Could you check a few things on this model? Use its own coordinates, in mm. A direction names the side the tool comes from. Round coordinates to 2 decimals unless told otherwise and drop trailing zeros. Loops run counter-clockwise (first coordinate to the right, second up) from the corner with the lowest first, then second, coordinate; pieces in that order, holes last. Notation, with made-up numbers: (-26.75, -33.75) - (-11.75, -33.75) arc R14 cw to (-11.75, -10.75) - close; hole circle Ø3 at (54.5, 28). An arc over 180 degrees is marked (long way). Answer as CSV lines item,"result". Start each with the question number.
1) We'd pull the mould along Z, two halves only. Please class faces 1 (the face through (0, -6.6, -6.1)), 2 (the face through (-2.17, -0.48, -7.53)), 3 (the face through (-5.714, 3.28, 18.811)): pulls with the +Z half, pulls with the -Z half, needs draft (parallel to the pull), parting line crosses it, or undercut.
2) Suppose I cut it at B-B, the plane z = -2.5. Write out the boundary of the cut face in (x, y), then the cut area to 3 significant figures.
3) I'm going to push flat-ended pins straight in: pin 1 Ø1.5 at (x, z) = (4, 10.5) entering from -Y; pin 2 Ø6 at (x, z) = (4.5, 4.5) entering from +Y; pin 3 Ø3 at (x, z) = (5, -13) entering from -Y; pin 4 Ø1.2 at (x, y) = (-1, 0) entering from +Z. Where does each tip first touch, or does it pass through?
4) Please list where these lines run through material, in increasing order: line 1 along Y through (x, z) = (0, 13.75); line 2 along Z through (x, y) = (2.25, 4); line 3 along Z through (x, y) = (1.5, -0.75).
5) Suppose I cut it at A-A, the plane z = 16.5. Write out the boundary of the cut face in (x, y).
6) Which directions (+Z, -Z, +X, -X, +Y, -Y) give clear straight access to the entire face, cutting with the end or side of a thin tool? Please do faces 4 (the face through (-5.7, 3.31, -6.11)), 5 (the face through (1.987, 0.626, 13.572)), 6 (the face through (3, 0, -6.35)), 7 (the face through (5.714, -3.28, 18.811)), 8 (the face through (-3.1, -0.69, -13.87)).
```python
from build123d import *

# Parameters (mm, degrees)
BOSS_EXTRUDE1_START = 19.05
BOSS_EXTRUDE1_DEPTH = 25.4
CHAMFER1_SIZE       = 0.9525
SKETCH4_R           = 2.0828
CUT_EXTRUDE1_DEPTH  = 11.1125
FILLET1_R           = 0.09921875
SKETCH5_OUTSIDE_W   = 101.45
SKETCH5_OUTSIDE_H   = 103.414
SKETCH5_OUTSIDE_R   = 6.35
CUT_EXTRUDE2_DEPTH  = 39.1
CUT_EXTRUDE2_TAPER  = 45
SKETCH6_OUTSIDE_W   = 76.05
SKETCH6_OUTSIDE_H   = 78.014
SKETCH6_OUTSIDE_R   = 6.35
CUT_EXTRUDE3_DEPTH  = 26.4
CUT_EXTRUDE3_TAPER  = 45


with BuildPart() as part:
    # Sketch2 → Boss-Extrude1 (new body)
    with BuildSketch(Plane.XY.offset(BOSS_EXTRUDE1_START)):
        Polygon((6.35, 3.666174209), (0, 7.332348419), (-6.35, 3.666174209), (-6.35, -3.666174209), (0, -7.332348419), (6.35, -3.666174209), align=None)
    extrude(amount=-BOSS_EXTRUDE1_DEPTH)

    # Sketch3 → Revolve1 (revolve)
    with BuildSketch(Plane(origin=(0, 0, 0), x_dir=(0, 0, -1), z_dir=(1, 0, 0))):
        Polygon((6.35, 2.2225), (8.5725, 2.2225), (9.525, 3.175), (19.05, 3.175), (19.05, 0), (6.35, 0), align=None)
    revolve(axis=Axis((0, 0, 19.05), (0, 0, -1)))

    # Chamfer1
    chamfer1_edges = [part.edges().sort_by_distance(p)[0] for p in [
        (0, -3.175, -19.05),
    ]]
    chamfer(chamfer1_edges, length=CHAMFER1_SIZE)

    # Sketch4 → Cut-Extrude1 (cut)
    with BuildSketch(Plane.XY.offset(19.05)):
        Circle(SKETCH4_R)
    extrude(amount=-CUT_EXTRUDE1_DEPTH, mode=Mode.SUBTRACT)

    # Fillet1
    fillet1_edges = [part.edges().sort_by_distance(p)[0] for p in [
        (0, -2.2225, -6.35),
    ]]
    fillet(fillet1_edges, radius=FILLET1_R)

    # Sketch5 outside → Cut-Extrude2 (cut, through all)
    with BuildSketch(Plane.XY.offset(19.05)):
        Rectangle(SKETCH5_OUTSIDE_W, SKETCH5_OUTSIDE_H)
        Circle(SKETCH5_OUTSIDE_R, mode=Mode.SUBTRACT)
    extrude(amount=-CUT_EXTRUDE2_DEPTH, taper=CUT_EXTRUDE2_TAPER, mode=Mode.SUBTRACT)

    # Sketch6 outside → Cut-Extrude3 (cut, through all)
    with BuildSketch(Plane(origin=(0, 0, -6.35), x_dir=(-1, 0, 0), z_dir=(0, 0, -1))):
        Rectangle(SKETCH6_OUTSIDE_W, SKETCH6_OUTSIDE_H)
        Circle(SKETCH6_OUTSIDE_R, mode=Mode.SUBTRACT)
    extrude(amount=-CUT_EXTRUDE3_DEPTH, taper=CUT_EXTRUDE3_TAPER, mode=Mode.SUBTRACT)


solid = part.part
```
Filled sheet:
1,face 1,"pulls with the -Z half"
1,face 2,"undercut"
1,face 3,"pulls with the +Z half"
2,outline,"(-6.35, -3.67) - (0, -7.33) - (6.35, -3.67) - (6.35, 3.67) - (0, 7.33) - (-6.35, 3.67) - close"
2,area,"140 mm²"
3,pin 1,"y = -5.46"
3,pin 2,"y = 6.47"
3,pin 3,"through"
3,pin 4,"z = 7.94"
4,line 1,"-7.33 to -2.08, 2.08 to 7.33"
4,line 2,"-6.35 to 19.05"
4,line 3,"-19.05 to 7.94"
5,outline,"(-6.35, -3.67) - (0, -7.33) - (6.35, -3.67) - (6.35, 3.67) - (0, 7.33) - (-6.35, 3.67) - close; hole circle Ø4.17 at (0, 0)"
6,face 4,"-Z, -X, +Y"
6,face 5,"+Z"
6,face 6,"none"
6,face 7,"+Z, +X, -Y"
6,face 8,"-Z"
